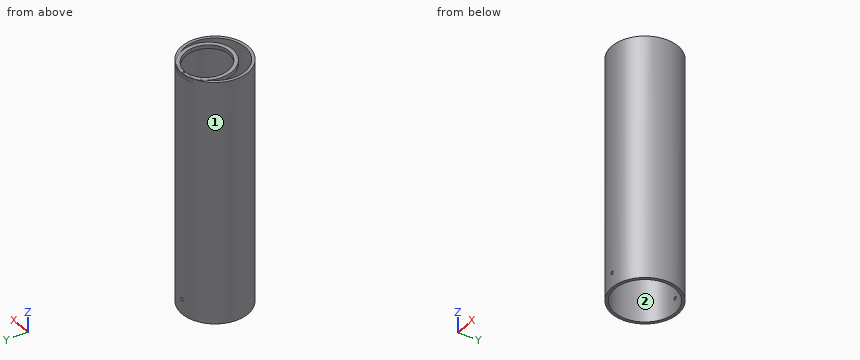
Autodesk Inventor part; units mm, degrees
ref_plane "Work Plane2" through (0, 45, 332) normal (0, 1, 0) x (-1, 0, 0)
ref_plane "Work Plane3" through (0, 41.1, 332) normal (0, 0.0605, 0.9982) x (1, 0, 0)
ref_plane "YZ Plane" through (0, 0, 0) normal (1, 0, 0) x (0, 1, 0)
sketch "Sketch1" plane through (0, 0, 0) normal (0, 0, 1) x (1, 0, 0)
  circle A0 centre (0, 0) radius 45
  circle A1 centre (0, 0) radius 41.1
  dimension "d0" = 90
  dimension "d2" = 3.9
extrude "Extrusion1" add sketch "Sketch1" along normal blind 332
sketch "Sketch2" plane through (0, 0, 332) normal (0, 0, 1) x (1, 0, 0)
  circle A0 centre (0, 0) radius 41.1
  circle A1 centre (0, 0) radius 45
  point P0 (0, 45)
ref_plane "Work Plane1" through (0, 45, 332) normal (0, 1, 0) x (-1, 0, 0)
sketch "Sketch5" plane through (0, 45, 332) normal (0, 1, 0) x (-1, 0, 0)
  circle A0 centre (0, -312) radius 4.4901
  point P0 (0, -332)
  dimension "d25" = 20
hole "nailHole" at (0, 45, 20) direction (0, -1, 0) diameter 4.5 end through all
sketch "Sketch6" plane through (0, 0, 332) normal (0, 0, 1) x (1, 0, 0)
  circle A0 centre (0, 0) radius 41.1
  circle A1 centre (0, 0) radius 45
  point P0 (0, 45)
ref_plane "Work Plane2" through (0, 45, 332) normal (0, 1, 0) x (-1, 0, 0)
sketch "Sketch10" plane through (0, 0, 332) normal (0, 0, 1) x (1, 0, 0)
  circle A0 centre (0, 0) radius 41.1
  circle A1 centre (0, 0) radius 45
  line L0 (0, 41.1) -> (46.8002, 41.1) construction
ref_plane "Work Plane3" through (0, 41.1, 332) normal (0, 0.0605, 0.9982) x (1, 0, 0)
sketch "Sketch11" plane through (0, 41.1, 332) normal (0, 0.0605, 0.9982) x (1, 0, 0)
  circle A0 centre (0, -30.1983) radius 30.1625
  circle A1 centre (0, -30.1983) radius 35.2425
  point P0 (0, -20.93)
  dimension "d44" = 60.325
  dimension "d45" = 5.08
extrude "INSERT_GUIDE_NOTFAB" add sketch "Sketch11" against normal blind 5.08
sketch "Sketch12" plane through (0, 41.1, 332) normal (0, 0.0605, 0.9982) x (1, 0, 0)
  circle A0 centre (0, -30.1983) radius 30.1625
  line L0 (-1.27, -0.4213) -> (1.27, -0.4213)
  line L1 (1.27, -0.4213) -> (1.27, 2.1187)
  line L2 (1.27, 2.1187) -> (-1.27, 2.1187)
  line L3 (-1.27, 2.1187) -> (-1.27, -0.4213)
  line L4 (0, 2.1187) -> (0, -0.4213) construction
  line L5 (0, -20.93) -> (0, -30.1983) construction
  dimension "d48" = 2.54
  dimension "d49" = 2.54
extrude "INSERT_KEY_NOTFAB" cut sketch "Sketch12" along normal mid plane 12.7 contours L1 L0 L3 A0 | A0 L3 L2 L1 picked at (0.1411, -0.2938)
sketch "Sketch14" plane through (0, 0, 332) normal (0, 0, 1) x (1, 0, 0)
  circle A0 centre (0, 0) radius 41.1
  line L0 (-6.35, 38.1) -> (6.35, 38.1)
  line L1 (0, 41.1) -> (0, 38.1) construction
  line L2 (-6.35, 38.1) -> (-6.35, 40.6065)
  line L3 (6.35, 38.1) -> (6.35, 40.6065)
  dimension "d52" = 12.7
  dimension "d53" = 3
extrude "shim" [suppressed]
equation "\"d0\" = sleeveOD"
equation "\"d2\" = sleeveWall"
equation "\"d3\" = sleeveLength"
equation "\"sleeveOD\" = 90"
equation "\"sleeveWall\" = 3.9"
equation "\"sleeveLength\" = 332"
equation "\"nailDelta\" = 20"
equation "\"sparLaunchAngle\" = 3.72deg"
properties part number "2h2slv" material "PVC-Piping"
Can you work these out from the model? Positions are in its coordinate system, mm. Face numbers are marked on the shaded views. Give positions to 0.01 mm unless a question says otherwise; leave off trailing zeros. Loops run counter-clockwise (first coordinate to the right, second up) from the corner with the lowest first, then second, coordinate; pieces in that order, holes last. Notation, with made-up numbers: M -10.75,-20 L 13.25,-20 A16 ccw 13.25,3 Z; hole C 13.25,40 d10. An arc over 180 degrees is marked long. One line per question, with ' | ' between items. Start each with the question number.
Q1. If we mould it in two halves opening along X, with no side actions, what happens to the marked faces 1 and 2? For each: +X half, -X half, draft (parallel to the pull), parting line (faces both ways), or undercut.
Q2. If we section it at C-C (y = 4): State how many separate pieces and enclosed holes the cut face has, plus the area to 3 significant figures.
Q3. If we section it at A-A (x = -8.5): Please give me the cut outline in (y, z).
Q4. If I drill on line 1 (X direction, y = 2, z = 282.5); line 2 (Y direction, x = 0, z = 135); line 3 (Z direction, x = 0, y = -43), over which ranges is the centre line in solid material (lowest first)? Write a range as from..to.
Q5. If we section it at B-B (z = 38): Please give me the cut outline in (x, y), plus the area to 3 significant figures.
Q6. For pin 1 Ø1.5 at (x, z) = (-4.5, 224) entering from -Y; pin 2 Ø2.5 at (y, z) = (41.5, 329) entering from +X; pin 3 Ø8 at (y, z) = (-29.5, 287) entering from -X; pin 4 Ø8 at (x, y) = (-14, 30) entering from +Z, each with a flat end and sliding along its axis, tell me the tip position at first contact or that it passes through.
Computed:
1) face 1: parting line | face 2: undercut
2) separate pieces: 4 | enclosed holes: 0 | area: 2,650 mm²
3) outline: M -44.19,0 L -40.21,0 L -40.21,332 L -44.19,332 Z; M -23.49,330.83 L -18.24,330.51 L -17.93,335.58 L -23.18,335.9 Z; M 39.54,327.01 L 40.21,326.96 L 40.21,0 L 44.19,0 L 44.19,326.72 L 44.79,326.69 L 45.1,331.76 L 44.19,331.81 L 44.19,332 L 41.1,332 L 39.84,332.08 Z
4) line 1: x = -44.96..-41.05, 41.05..44.96 | line 2: y = -45..-41.1, 41.1..45 | line 3: z = 0..17.75, 22.25..332
5) outline: C 0,0 d90; hole C 0,0 d82.2 | area: 1,050 mm²
6) pin 1: stops at y = -44.84 | pin 2: stops at x = 20.12 | pin 3: stops at x = -37.08 | pin 4: passes through
